Work out the finished part from the listing and answer in its coordinate system (mm). Face numbers are marked on the shaded views. A direction names the side the tool comes from. Round coordinates to 2 decimals unless told otherwise and drop trailing zeros. Loops run counter-clockwise (first coordinate to the right, second up) from the corner with the lowest first, then second, coordinate; pieces in that order, holes last. Notation, with made-up numbers: (-30, -27.5) -> (9, -27.5) arc R29 ccw to (9, 2.5) -> close; hole circle Ø8 at (23, -13.75). An arc over 180 degrees is marked (long way). Use one line per item in the form item = value.
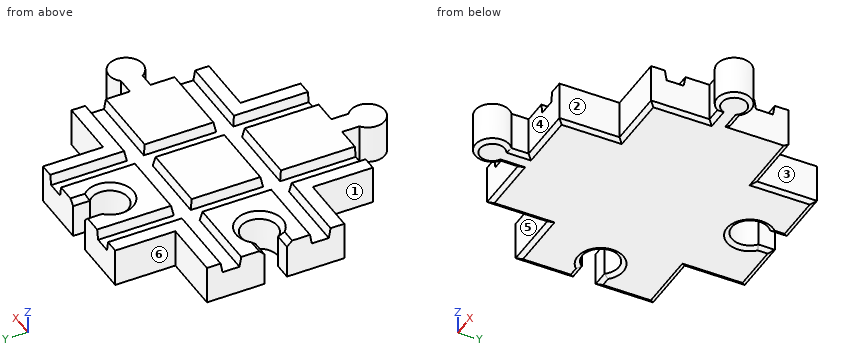
```python
from build123d import *

# Parameters (mm, degrees)
F0_W      = 40
F0_H      = 12
F1_DEPTH  = 75
F3_DEPTH  = 12
F5_DEPTH  = 12
F7_DEPTH  = 75
F9_DEPTH  = 75
F10_SIZE2 = 0.8
F10_SIZE  = 1.3856406461
F11_SIZE  = 1.5


with BuildPart() as f1:
    # F0 (on Right) → F1 (new body)
    with BuildSketch(Plane.YZ):
        with Locations((0, 6)):
            Rectangle(F0_W, F0_H)
    extrude(amount=F1_DEPTH)

    # F2 (on face) → F3 (join)
    with BuildSketch(Plane.XY.offset(12)):
        with BuildLine():
            Line((40.5, -37.5), (57.5, -37.5))
            Line((57.5, -37.5), (57.5, 37.5))
            Line((57.5, 37.5), (40.8, 37.5))
            Line((40.8, 37.5), (40.8, 32.6472882707))
            ThreePointArc((40.8, 32.6472882707), (37.5, 23.2), (34.2, 32.6472882707))
            Line((34.2, 32.6472882707), (34.2, 37.5))
            Line((34.2, 37.5), (17.5, 37.5))
            Line((17.5, 37.5), (17.5, -37.5))
            Line((17.5, -37.5), (34.5, -37.5))
            Line((34.5, -37.5), (34.5, -42.5))
            ThreePointArc((34.5, -42.5), (37.5, -51.5), (40.5, -42.5))
            Line((40.5, -42.5), (40.5, -37.5))
        make_face()
        with BuildLine():
            Line((80, 3), (75, 3))
            Line((75, 3), (75, -3))
            Line((75, -3), (79.4055112535, -3))
            ThreePointArc((79.4055112535, -3), (88.6478954729, -0.8862974958), (80, 3))
        make_face()
    extrude(amount=-F3_DEPTH)

    # F4 (on face) → F5 (cut)
    with BuildSketch(Plane.XY.offset(12)):
        with BuildLine():
            Line((0, 3.3), (0, 3))
            Line((0, 3), (0, -3))
            Line((0, -3), (0, -3.3))
            Line((0, -3.3), (4.8527117293, -3.3))
            ThreePointArc((4.8527117293, -3.3), (14.3, 0), (4.8527117293, 3.3))
            Line((4.8527117293, 3.3), (0, 3.3))
        make_face()
    extrude(amount=-F5_DEPTH, mode=Mode.SUBTRACT)

    # F6 (on face) → F7 (cut)
    with BuildSketch(Plane.YZ.offset(75)):
        Polygon((-10, 12), (-16, 12), (-15.4710190579, 9), (-10.5289809421, 9), align=None)
        Polygon((15.4710190579, 9), (16, 12), (10, 12), (10.5289809421, 9), align=None)
    extrude(amount=-F7_DEPTH, mode=Mode.SUBTRACT)

    # F8 (on face) → F9 (cut)
    with BuildSketch(Plane(origin=(0, 37.5, 0), x_dir=(-1, 0, 0), z_dir=(0, 1, 0))):
        Polygon((-47.5, 12), (-53.5, 12), (-52.9710190579, 9), (-48.0289809421, 9), align=None)
        Polygon((-21.5, 12), (-27.5, 12), (-26.9710190579, 9), (-22.0289809421, 9), align=None)
    extrude(amount=-F9_DEPTH, mode=Mode.SUBTRACT)

    # F10
    f10_edges = [f1.edges().sort_by_distance(p)[0] for p in [
        (37.5, -51.5, 0),
        (40.5, -40, 0),
        (49, -37.5, 0),
        (66.25, -20, 0),
        (34.5, -40, 0),
        (75, -11.5, 0),
        (57.5, -28.75, 0),
        (77.5, 3, 0),
        (77.202756, -3, 0),
        (88.647895, -0.886297, 0),
        (66.25, 20, 0),
        (57.5, 28.75, 0),
        (49.15, 37.5, 0),
        (40.8, 35.073644, 0),
        (37.5, 23.2, 0),
        (34.2, 35.073644, 0),
        (25.85, 37.5, 0),
        (17.5, 28.75, 0),
        (8.75, 20, 0),
        (2.426356, -3.3, 0),
        (14.3, 0, 0),
        (2.426356, 3.3, 0),
        (0, 11.65, 0),
        (0, -11.65, 0),
        (8.75, -20, 0),
        (17.5, -28.75, 0),
        (26, -37.5, 0),
    ]]
    f10_side = f1.faces().sort_by_distance((39.337765, -1.867927, 0))[0]
    chamfer(f10_edges, length=F10_SIZE, length2=F10_SIZE2, reference=f10_side)

    # F11
    f11_edges = [f1.edges().sort_by_distance(p)[0] for p in [
        (2.426356, -3.3, 12),
        (14.3, 0, 12),
        (2.426356, 3.3, 12),
        (37.5, 23.2, 12),
        (34.2, 35.073644, 12),
        (40.8, 35.073644, 12),
    ]]
    chamfer(f11_edges, length=F11_SIZE)


solid = f1.part
```
(1) Find section D-D, the plane x = 37.5. Write down the section's boundary in (y, z), then the cut area to 3 significant figures.
Completed:
outline = (-51.5, 0.8) -> (-50.11, 0) -> (21.81, 0) -> (23.2, 0.8) -> (23.2, 10.5) -> (21.7, 12) -> (16, 12) -> (15.47, 9) -> (10.53, 9) -> (10, 12) -> (-10, 12) -> (-10.53, 9) -> (-15.47, 9) -> (-16, 12) -> (-51.5, 12) -> close
area = 861 mm2
(2) Given P1, Ø3.5, axis at y = 28, z = 5, coming from the +X side; P2, Ø5.5, axis at x = 1.5, z = 6, coming from the -Y side; P3, Ø2.5, axis at y = -40, z = 5, coming from the -X side, each flat-ended and moving along its own axis, determine where each tip first touches the part or whether it passes through.
Completed:
P1 = 57.5
P2 = -20
P3 = 34.5
(3) Find section C-C, the plane z = 2. Write down the section's boundary in (x, y), then the cut area to 3 significant figures.
Completed:
outline = (0, -20) -> (17.5, -20) -> (17.5, -37.5) -> (34.5, -37.5) -> (34.5, -42.5) arc R5 ccw (long way) to (40.5, -42.5) -> (40.5, -37.5) -> (57.5, -37.5) -> (57.5, -20) -> (75, -20) -> (75, -3) -> (79.41, -3) arc R5 ccw (long way) to (80, 3) -> (75, 3) -> (75, 20) -> (57.5, 20) -> (57.5, 37.5) -> (40.8, 37.5) -> (40.8, 32.65) arc R5.3 cw (long way) to (34.2, 32.65) -> (34.2, 37.5) -> (17.5, 37.5) -> (17.5, 20) -> (0, 20) -> (0, 3.3) -> (4.85, 3.3) arc R5.3 cw (long way) to (4.85, -3.3) -> (0, -3.3) -> close
area = 4,380 mm2
(4) Consider L1, parallel to X at y = 28.5, z = 5; L2, parallel to Y at x = 46, z = 10.5; L3, parallel to X at y = 33.5, z = 5.5. Determine where each line is inside the solid, lowest interval first.
Completed:
L1 = 17.5 to 32.2, 42.8 to 57.5
L2 = -37.5 to -15.74, -10.26 to 10.26, 15.74 to 37.5
L3 = 17.5 to 34.2, 40.8 to 57.5
(5) Find section A-A, the plane x = 9. Write down the section's boundary in (y, z), then the cut area to 3 significant figures.
Completed:
outline = (-20, 0.8) -> (-18.61, 0) -> (-6.69, 0) -> (-5.3, 0.8) -> (-5.3, 10.5) -> (-6.8, 12) -> (-10, 12) -> (-10.53, 9) -> (-15.47, 9) -> (-16, 12) -> (-20, 12) -> close; (5.3, 0.8) -> (6.69, 0) -> (18.61, 0) -> (20, 0.8) -> (20, 12) -> (16, 12) -> (15.47, 9) -> (10.53, 9) -> (10, 12) -> (6.8, 12) -> (5.3, 10.5) -> close
area = 316 mm2
(6) For a pull along Y with two mould halves and no side action, classify the marked faces 4, 5 and 6 as +Y half, -Y half, draft (parallel to the pull), parting line (faces both ways), or undercut.
Completed:
face_4 = undercut
face_5 = -Y half
face_6 = draft
(7) For the marked faces 1, 2 and 3, determine the directions among +Z, -Z, +X, -X, +Y, -Y from which every point of the face is accessible in a straight line to the end or side of a thin tool.
Completed:
face_1 = +Z, -Z, -X, -Y
face_2 = +Z, -Z, +X, -Y
face_3 = +Z, -Z, +X, +Y
(8) Find section B-B, the plane y = 28.5. Write down the section's boundary in (x, z), then the cut area to 3 significant figures.
Completed:
outline = (17.5, 0.8) -> (18.89, 0) -> (30.81, 0) -> (32.2, 0.8) -> (32.2, 10.5) -> (30.7, 12) -> (27.5, 12) -> (26.97, 9) -> (22.03, 9) -> (21.5, 12) -> (17.5, 12) -> close; (42.8, 0.8) -> (44.19, 0) -> (56.11, 0) -> (57.5, 0.8) -> (57.5, 12) -> (53.5, 12) -> (52.97, 9) -> (48.03, 9) -> (47.5, 12) -> (44.3, 12) -> (42.8, 10.5) -> close
area = 316 mm2
